from build123d import *

# Parameters (mm, degrees)
PAD020_DEPTH    = 7
SKETCH043_W     = 30
SKETCH043_H     = 11.8536046546
POCKET018_DEPTH = 2.5
SKETCH044_R     = 1.5
POCKET019_DEPTH = 10
SKETCH045_R     = 3.5
POCKET020_DEPTH = 3
SKETCH046_R     = 18.15
POCKET021_DEPTH = 10
POCKET022_DEPTH = 2.5


with BuildPart() as part:
    # Sketch042 → Pad020 (new body)
    with BuildSketch(Plane.XY):
        Polygon((-12.8493066257, -33.7940933811), (-8.2452066191, -2.9618052463), (0.8857658642, 11.8536046546), (29.1142341358, 11.8536046546), (38.335521046, -2.8996050949), (42.948959357, -33.794429076), (33.0593993066, -35.2712096281), (28.4644789539, -4.5003949051), (23.3502319582, 3.6819292513), (6.6497680418, 3.6819292513), (1.6452066191, -4.4381947537), (-2.9589691174, -35.2709900288), align=None)
    extrude(amount=PAD020_DEPTH)

    # Sketch043 (on Face13 of Pad020) → Pocket018 (cut)
    with BuildSketch(Plane(origin=(0, 0, 0), x_dir=(1, 0, 0), z_dir=(0, 0, -1))):
        with Locations((15, -5.9268023273)):
            Rectangle(SKETCH043_W, SKETCH043_H)
    extrude(amount=-POCKET018_DEPTH, mode=Mode.SUBTRACT)

    # Sketch044 (on Face5 of Pocket018) → Pocket019 (cut)
    with BuildSketch(Plane.XY.offset(7)):
        with Locations((3.767766953, 7.767766953)):
            Circle(SKETCH044_R)
        with Locations((26.232233047, 7.767766953)):
            Circle(SKETCH044_R)
        with Locations((-6.8703102168, -27.60930544)):
            Circle(SKETCH044_R)
        with Locations((36.9703102168, -27.60930544)):
            Circle(SKETCH044_R)
        with Locations((33.4, -3.7)):
            Circle(SKETCH044_R)
        with Locations((-3.3, -3.7)):
            Circle(SKETCH044_R)
    extrude(amount=-POCKET019_DEPTH, mode=Mode.SUBTRACT)

    # Sketch045 (on Face5 of Pocket019) → Pocket020 (cut)
    with BuildSketch(Plane.XY.offset(7)):
        with Locations((36.9703102168, -27.60930544)):
            Circle(SKETCH045_R)
        with Locations((33.4, -3.7)):
            Circle(SKETCH045_R)
        with Locations((26.232233047, 7.767766953)):
            Circle(SKETCH045_R)
        with Locations((3.767766953, 7.767766953)):
            Circle(SKETCH045_R)
        with Locations((-3.3, -3.7)):
            Circle(SKETCH045_R)
        with Locations((-6.8703102168, -27.60930544)):
            Circle(SKETCH045_R)
    extrude(amount=-POCKET020_DEPTH, mode=Mode.SUBTRACT)

    # Sketch046 (on Face5 of Pocket020) → Pocket021 (cut)
    with BuildSketch(Plane.XY.offset(7)):
        with Locations((15.05, -27.60930544)):
            Circle(SKETCH046_R)
    extrude(amount=-POCKET021_DEPTH, mode=Mode.SUBTRACT)

    # Sketch047 (on Face4 of Pocket021) → Pocket022 (cut)
    with BuildSketch(Plane(origin=(0, 0, 0), x_dir=(1, 0, 0), z_dir=(0, 0, -1))):
        with BuildLine():
            ThreePointArc((-8.3120846255, 30.7022032745), (-10.3000000009, 27.6093139691), (-8.3121001429, 24.5164146902))
            Line((-8.3121001429, 24.5164146902), (-2.5265008251, 21.8749228678))
            Line((-2.5265008251, 21.8749228678), (32.6264961364, 21.8749207273))
            Line((38.4120727539, 24.5164021866), (32.6264961364, 21.8749207273))
            ThreePointArc((38.4120727539, 24.5164021867), (40.3999999994, 27.6092903858), (38.4121001427, 30.7021961887))
            Line((32.6265008251, 33.3436880121), (38.4121001427, 30.7021961887))
            Line((-2.5265008251, 33.3436880122), (32.6265008251, 33.3436880121))
            Line((-8.3120846255, 30.7022032745), (-2.5265008251, 33.3436880122))
        make_face()
    extrude(amount=-POCKET022_DEPTH, mode=Mode.SUBTRACT)


with BuildPart() as part_1:
    # Body005 placement: moved
    add(part.part.moved(Location((0, 0, 2.5))))


solid = part_1.part
Geometry: final body of the model. Coordinates: model frame, mm. A direction names the side the tool comes from. Give positions to 0.01 mm unless a question says otherwise; leave off trailing zeros. Order: outer loops, then holes, each group sorted by start corner. A loop starts at its lowest first (then second) coordinate and runs counter-clockwise, first axis right, second up. Notation, with made-up numbers: (58, -10) -> (72, -10) arc R4 ccw to (72, -3) -> close; hole circle Ø9 at (61.5, -20.75). An arc over 180 degrees is marked (long way). Answer as a JSON object with one key per item and string values.
Q1. First-contact query: pin 1 (2.5 mm diameter, centred on x = 38, y = -28.5, fed in from -Z); pin 2 (1.2 mm diameter, centred on y = 4.5, z = 4, fed in from +X); pin 3 (1.5 mm diameter, centred on y = -27, z = 4.5, fed in from +X); pin 4 (2 mm diameter, centred on x = 16, z = 3.5, fed in from -Y). Flat tips, straight axial feed; report the tip coordinate or a pass-through.
Entries:
{"pin 1": "stops at z = 5", "pin 2": "stops at x = 34.09", "pin 3": "stops at x = 42.05", "pin 4": "passes through"}
Q2. Section C-C (x = 19.5). Output: boundary loops of the cut face in (y, z), plus the area to 3 significant figures.
Entries:
{"outline": "(3.68, 5) -> (11.85, 5) -> (11.85, 9.5) -> (3.68, 9.5) -> close", "area": "36.8 mm^2"}
Q3. Draft query along X for faces 6 (the flat face through (38, -29, 6.5)), 7 (the flat face through (-7.835, -34.543, 5.951)), 8 (the flat face through (-4, -12, 2.5)), 9 (the flat face through (38.073, -34.522, 5.951)). Return one class per face: released by +X, released by -X, zero draft, split by the parting line, or undercut.
Entries:
{"face 6": "undercut", "face 7": "released by -X", "face 8": "zero draft", "face 9": "released by +X"}
Q4. Material intervals for probe 1 along X at (y, z) = (-1, 7.5); probe 2 along Z at (x, y) = (33, -7); probe 3 along X at (y, z) = (-3, 6), sorted ascending.
Entries:
{"probe 1": "x = -7.04 to -5.53, -1.07 to 3.76, 26.28 to 31.17, 35.63 to 37.15", "probe 2": "z = 2.5 to 6.5", "probe 3": "x = -8.25 to -4.63, -1.97 to 2.53, 27.53 to 32.07, 34.73 to 38.35"}
Q5. Access query for faces 1 (the flat face through (15, 11.854, 7)), 2 (the cylindrical face through (23.455, 5.638, 8.021)), 3 (the flat face through (35, -28, 5)), 4 (the flat face through (30, 5, 4)), 5 (the flat face through (34, -12, 2.5)). Directions: +Z, -Z, +X, -X, +Y, -Y. A direction counts if a zero-diameter tool reaches every point of the face in a straight line with its end or side. Return the directions, or none.
Entries:
{"face 1": "+Z, -Z, +X, -X, +Y", "face 2": "+Z", "face 3": "-Z", "face 4": "-Z, +Y", "face 5": "-Z, +X, -X, +Y, -Y"}
Q6. Section D-D (z = 7.5). Output: boundary loops of the cut face in (x, y).
Entries:
{"outline": "(-12.85, -33.79) -> (-2.96, -35.27) -> (-2.5, -32.22) arc R18.15 cw to (-0.39, -18.07) -> (1.65, -4.44) -> (6.65, 3.68) -> (23.35, 3.68) -> (28.46, -4.5) -> (30.49, -18.07) arc R18.15 cw to (32.6, -32.22) -> (33.06, -35.27) -> (42.95, -33.79) -> (38.34, -2.9) -> (29.11, 11.85) -> (0.89, 11.85) -> (-8.25, -2.96) -> close; hole circle Ø7 at (-6.87, -27.61); hole circle Ø7 at (-3.3, -3.7); hole circle Ø7 at (3.77, 7.77); hole circle Ø7 at (26.23, 7.77); hole circle Ø7 at (33.4, -3.7); hole circle Ø7 at (36.97, -27.61)"}
Q7. Section B-B (y = -3.7). Output: boundary loops of the cut face in (x, z), plus the area to 3 significant figures.
Entries:
{"outline": "(-8.36, 2.5) -> (-4.8, 2.5) -> (-4.8, 6.5) -> (-6.8, 6.5) -> (-6.8, 9.5) -> (-8.36, 9.5) -> close; (-1.8, 2.5) -> (2.1, 2.5) -> (2.1, 9.5) -> (0.2, 9.5) -> (0.2, 6.5) -> (-1.8, 6.5) -> close; (27.96, 2.5) -> (31.9, 2.5) -> (31.9, 6.5) -> (29.9, 6.5) -> (29.9, 9.5) -> (27.96, 9.5) -> close; (34.9, 2.5) -> (38.46, 2.5) -> (38.46, 9.5) -> (36.9, 9.5) -> (36.9, 6.5) -> (34.9, 6.5) -> close", "area": "80.6 mm^2"}
Q8. Section A-A (z = 4). Output: boundary loops of the cut face in (x, y).
Entries:
{"outline": "(-12.85, -33.79) -> (-2.96, -35.27) -> (-2.66, -33.28) -> (-8.31, -30.7) arc R3.4 cw to (-8.31, -24.52) -> (-2.53, -21.87) -> (-2.17, -21.87) arc R18.15 cw to (-0.39, -18.07) -> (1.65, -4.44) -> (4.38, 0) -> (0, 0) -> (0, 10.42) -> (-8.25, -2.96) -> close; (25.65, 0) -> (28.46, -4.5) -> (30.49, -18.07) arc R18.15 cw to (32.27, -21.87) -> (32.63, -21.87) -> (38.41, -24.52) arc R3.4 cw to (38.41, -30.7) -> (32.76, -33.28) -> (33.06, -35.27) -> (42.95, -33.79) -> (38.34, -2.9) -> (30, 10.44) -> (30, 0) -> close; hole circle Ø3 at (-3.3, -3.7); hole circle Ø3 at (33.4, -3.7)"}
